Read the model definition and answer for the solid it produces. Units are mm, in the model's axes. A direction names the side the tool comes from. Give positions to 0.01 mm unless a question says otherwise; leave off trailing zeros. Loops run counter-clockwise (first coordinate to the right, second up) from the corner with the lowest first, then second, coordinate; pieces in that order, holes last. Notation, with made-up numbers: (-24, 86) - (-8, 86) arc R21 ccw to (-8, 106) - close; hole circle Ø10 at (-19, 49). An arc over 180 degrees is marked (long way). Write item = value, one per line. Start each with the question number.
from build123d import *

# Parameters (mm, degrees)
BOX044_W      = 181
BOX044_H      = 122.4
BOX044_DEPTH  = 10
BOX045_W      = 184
BOX045_H      = 125.4
BOX045_DEPTH  = 10
FILLET005_1_R = 3
FILLET005_2_R = 1


with BuildPart() as cube022:
    # Box044 → Box044 (new body)
    with BuildSketch(Plane(origin=(-0.2, -0.2, 0), x_dir=(1, 0, 0), z_dir=(0, 0, 1))):
        with Locations((90.5, 61.2)):
            Rectangle(BOX044_W, BOX044_H)
    extrude(amount=BOX044_DEPTH)


with BuildPart() as fillet005:
    # Box045 → Box045 (new body)
    with BuildSketch(Plane(origin=(-1.5, -1.5, -1), x_dir=(1, 0, 0), z_dir=(0, 0, 1))):
        with Locations((92, 62.7)):
            Rectangle(BOX045_W, BOX045_H)
    extrude(amount=BOX045_DEPTH)

    # Cut007: cut Cube022
    add(cube022.part, mode=Mode.SUBTRACT)

    # Fillet005 1
    fillet005_1_edges = [fillet005.edges().sort_by_distance(p)[0] for p in [
        (-1.5, -1.5, 4),
        (-1.5, 123.9, 4),
        (182.5, -1.5, 4),
        (182.5, 123.9, 4),
    ]]
    fillet(fillet005_1_edges, radius=FILLET005_1_R)

    # Fillet005 2
    fillet005_2_edges = [fillet005.edges().sort_by_distance(p)[0] for p in [
        (180.8, -0.2, 4.5),
        (-0.2, -0.2, 4.5),
        (180.8, 122.2, 4.5),
        (-0.2, 122.2, 4.5),
    ]]
    fillet(fillet005_2_edges, radius=FILLET005_2_R)


solid = fillet005.part
1. Consider line 1 along Y through (x, z) = (19, 0.5); line 2 along X through (y, z) = (106, 5); line 3 along Z through (x, y) = (15, 100). Determine where each line is inside the solid, lowest interval first. Write a range as [from, to].
2. For a pull along X with two mould halves and no side action, classify faces 3 (the flat face through (89, 123.9, 4)), 4 (the flat face through (-1.5, 60, 4)), 5 (the flat face through (180.8, 60, 4)) as released by +X, released by -X, zero draft, split by the parting line, or undercut.
3. A tool of negligible diameter and unlimited length cuts with its end or side. For faces 1 (the flat face through (-0.2, 60, 4)), 2 (the flat face through (89, 62, -1)), from which of +Z, -Z, +X, -X, +Y, -Y can it reach the whole face along a straight path? Write none if from no direction.
4. A cutting plane is placed at B-B on x = 154.5. Give the vertices of the cut face in (y, z), and give its area (3 significant figures).
5. A cutting plane is placed at A-A on z = 5. Give the vertices of the cut face in (x, y).
6. Given P1, Ø4, axis at x = 53, y = 99, coming from the +Z side, flat-ended and moving along its own axis, determine where the tip first touches the part or whether it passes through.
7. A cutting plane is placed at C-C on y = 103. Give the vertices of the cut face in (x, z), and give its area (3 significant figures).
Reply:
q1.line_1 = [-1.5, -0.2], [122.2, 123.9]
q1.line_2 = [-1.5, -0.2], [180.8, 182.5]
q1.line_3 = [-1, 0]
q2.face_3 = zero draft
q2.face_4 = released by -X
q2.face_5 = undercut
q3.face_1 = +Z
q3.face_2 = -Z, +X, -X, +Y, -Y
q4.outline = (-1.5, -1) - (123.9, -1) - (123.9, 9) - (122.2, 9) - (122.2, 0) - (-0.2, 0) - (-0.2, 9) - (-1.5, 9) - close
q4.area = 152 mm^2
q5.outline = (-1.5, 1.5) arc R3 ccw to (1.5, -1.5) - (179.5, -1.5) arc R3 ccw to (182.5, 1.5) - (182.5, 120.9) arc R3 ccw to (179.5, 123.9) - (1.5, 123.9) arc R3 ccw to (-1.5, 120.9) - close; hole (-0.2, 0.8) arc R1 ccw to (0.8, -0.2) - (179.8, -0.2) arc R1 ccw to (180.8, 0.8) - (180.8, 121.2) arc R1 ccw to (179.8, 122.2) - (0.8, 122.2) arc R1 ccw to (-0.2, 121.2) - close
q6.P1 = 0
q7.outline = (-1.5, -1) - (182.5, -1) - (182.5, 9) - (180.8, 9) - (180.8, 0) - (-0.2, 0) - (-0.2, 9) - (-1.5, 9) - close
q7.area = 211 mm^2
